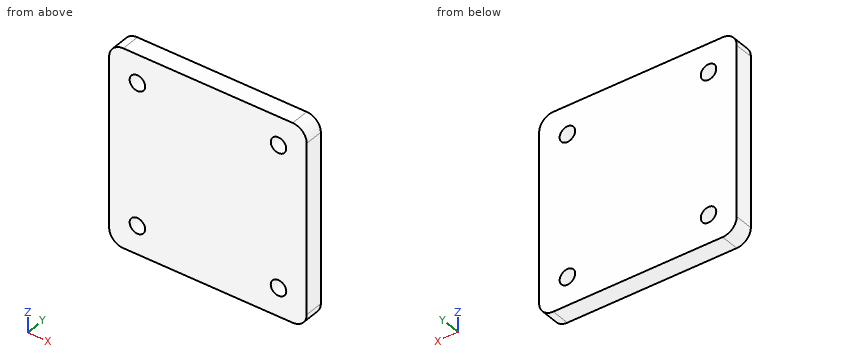
```python
from build123d import *

# Parameters (mm, degrees)
SKETCH_1_W          = 42
SKETCH_1_H          = 4
BLOCKEXTRUDE_DEPTH  = 42
FILLET_2_R          = 3
SKETCH_2_R          = 1.65
MOUNT_HOLE_DEPTH    = 60.531504265
SKETCH_3_R          = 1.65
CUT_EXTRUDE_2_DEPTH = 60.531504265
SKETCH_4_R          = 1.65
CUT_EXTRUDE_3_DEPTH = 60.531504265
SKETCH_5_R          = 1.65
CUT_EXTRUDE_4_DEPTH = 60.531504265


with BuildPart() as part:
    # 草图1 → BlockExtrude (new body)
    with BuildSketch(Plane.XY):
        with Locations((21, 2)):
            Rectangle(SKETCH_1_W, SKETCH_1_H)
    extrude(amount=BLOCKEXTRUDE_DEPTH)

    # Fillet 2
    fillet_2_edges = [part.edges().sort_by_distance(p)[0] for p in [
        (42, 2, 42),
        (0, 2, 42),
        (42, 2, 0),
        (0, 2, 0),
    ]]
    fillet(fillet_2_edges, radius=FILLET_2_R)

    # 草图2 → Mount_hole (cut, through all)
    with BuildSketch(Plane(origin=(0, 4, 0), x_dir=(1, 0, 0), z_dir=(0, 1, 0))):
        with Locations(Location((6, -6, 0), (0, 0, 270))):
            Circle(SKETCH_2_R)
    extrude(amount=-MOUNT_HOLE_DEPTH, mode=Mode.SUBTRACT)

    # 草图3 → 切除-拉伸2 (cut, through all)
    with BuildSketch(Plane(origin=(0, 4, 0), x_dir=(1, 0, 0), z_dir=(0, 1, 0))):
        with Locations(Location((6, -36, 0), (0, 0, 270))):
            Circle(SKETCH_3_R)
    extrude(amount=-CUT_EXTRUDE_2_DEPTH, mode=Mode.SUBTRACT)

    # 草图4 → 切除-拉伸3 (cut, through all)
    with BuildSketch(Plane(origin=(0, 4, 0), x_dir=(1, 0, 0), z_dir=(0, 1, 0))):
        with Locations(Location((36, -6, 0), (0, 0, 270))):
            Circle(SKETCH_4_R)
    extrude(amount=-CUT_EXTRUDE_3_DEPTH, mode=Mode.SUBTRACT)

    # 草图5 → 切除-拉伸4 (cut, through all)
    with BuildSketch(Plane(origin=(0, 4, 0), x_dir=(1, 0, 0), z_dir=(0, 1, 0))):
        with Locations(Location((36, -36, 0), (0, 0, 270))):
            Circle(SKETCH_5_R)
    extrude(amount=-CUT_EXTRUDE_4_DEPTH, mode=Mode.SUBTRACT)


solid = part.part
```
The listing builds one solid part. Answer for the finished solid, in the listing's coordinates (mm). Round coordinates to 2 decimals unless told otherwise and drop trailing zeros. Loops run counter-clockwise (first coordinate to the right, second up) from the corner with the lowest first, then second, coordinate; pieces in that order, holes last. Notation, with made-up numbers: (-38.75, 2) - (19.25, 2) arc R31 ccw to (19.25, 30) - close; hole circle Ø1 at (67, -39). An arc over 180 degrees is marked (long way). Return JSON: item names as keys, results as strings. Group by question number.
1. The part is cut by section C-C on y = 1.1. Determine the outline of the cut face in (x, z).
2. The part is cut by section A-A on x = 6. Determine the outline of the cut face in (y, z).
3. Each of these flat-tipped pins is pushed along its axis until it touches: P1, Ø5.5, axis at x = 6, z = 6, coming from the +Y side; P2, Ø2.5, axis at x = 36, z = 6, coming from the +Y side. Where does it stop, or does it pass through?
4. The part is cut by section B-B on z = 6. Determine the outline of the cut face in (x, y), then the cut area to 3 significant figures.
5. Consider probe 1 along X at (y, z) = (2.1, 6); probe 2 along Z at (x, y) = (7, 2.25); probe 3 along Z at (x, y) = (7.5, 3.3). Determine where each line is inside the solid, lowest interval first.
Resolved:
{
 "1": {"outline": "(0, 3) arc R3 ccw to (3, 0) - (39, 0) arc R3 ccw to (42, 3) - (42, 39) arc R3 ccw to (39, 42) - (3, 42) arc R3 ccw to (0, 39) - close; hole circle Ø3.3 at (6, 6); hole circle Ø3.3 at (6, 36); hole circle Ø3.3 at (36, 6); hole circle Ø3.3 at (36, 36)"},
 "2": {"outline": "(0, 0) - (4, 0) - (4, 4.35) - (0, 4.35) - close; (0, 7.65) - (4, 7.65) - (4, 34.35) - (0, 34.35) - close; (0, 37.65) - (4, 37.65) - (4, 42) - (0, 42) - close"},
 "3": {"P1": "stops at y = 4", "P2": "passes through"},
 "4": {"outline": "(0, 0) - (4.35, 0) - (4.35, 4) - (0, 4) - close; (7.65, 0) - (34.35, 0) - (34.35, 4) - (7.65, 4) - close; (37.65, 0) - (42, 0) - (42, 4) - (37.65, 4) - close", "area": "142 mm²"},
 "5": {"probe 1": "x = 0 to 4.35, 7.65 to 34.35, 37.65 to 42", "probe 2": "z = 0 to 4.69, 7.31 to 34.69, 37.31 to 42", "probe 3": "z = 0 to 5.31, 6.69 to 35.31, 36.69 to 42"}
}
